Geometry check sheet. Reference: the model listing, model coordinates, mm. Round coordinates to 2 decimals unless told otherwise and drop trailing zeros. One line per item, written item: value. Start each with the question number.
1. Section check A-A (x = 225). Count the separate pieces of the cut face and the enclosed holes in it, and give its area (3 significant figures).
2. Depth check by flat-ended pin: P1, Ø4, axis at x = 245.5, z = -114, coming from the +Y side. Enter the tip coordinate at first touch or a pass-through.
3. Scan lines: probe 1 along Z at (x, y) = (234, 4.2); probe 2 along X at (y, z) = (2.5, -82.5); probe 3 along X at (y, z) = (9.2, -94.25). Record each from-to range of solid material in increasing order. Write a range as [from, to].
from build123d import *

# Parameters (mm, degrees)
SKICA1_W                 = 400
SKICA1_H                 = 225
P_IDAT_VYSUNUT_M1_DEPTH  = 10
SKICA2_R                 = 102.5
ODEBRAT_VYSUNUT_M1_DEPTH = 10
ZAOBLIT1_R               = 10
SKICA3_R                 = 4
ODEBRAT_VYSUNUT_M2_DEPTH = 10
SKICA4_R                 = 7.5
ODEBRAT_VYSUNUT_M3_DEPTH = 6
ZKOSEN_1_SIZE            = 0.5
ZKOSEN_2_SIZE            = 1
ZKOSEN_3_SIZE            = 1
SKICA5_R                 = 2
ODEBRAT_VYSUNUT_M4_DEPTH = 10
SKICA6_R                 = 2
ODEBRAT_VYSUNUT_M5_DEPTH = 10
SKICA7_R                 = 4
ODEBRAT_VYSUNUT_M6_DEPTH = 4


with BuildPart() as part:
    # Skica1 → Přidat vysunutím1 (new body)
    with BuildSketch(Plane(origin=(0, 0, 0), x_dir=(1, 0, 0), z_dir=(0, 1, 0))):
        with Locations((200, 112.5)):
            Rectangle(SKICA1_W, SKICA1_H)
    extrude(amount=P_IDAT_VYSUNUT_M1_DEPTH)

    # Skica2 → Odebrat vysunutím1 (cut)
    with BuildSketch(Plane(origin=(0, 10, 0), x_dir=(1, 0, 0), z_dir=(0, 1, 0))):
        with Locations(Location((112.5, 112.5, 0), (0, 0, 270))):
            Circle(SKICA2_R)
    extrude(amount=-ODEBRAT_VYSUNUT_M1_DEPTH, mode=Mode.SUBTRACT)

    # Zaoblit1
    zaoblit1_edges = [part.edges().sort_by_distance(p)[0] for p in [
        (0, 5, -225),
        (400, 5, -225),
        (400, 5, 0),
        (0, 5, 0),
    ]]
    fillet(zaoblit1_edges, radius=ZAOBLIT1_R)

    # Skica3 → Odebrat vysunutím2 (cut)
    with BuildSketch(Plane(origin=(0, 10, 0), x_dir=(1, 0, 0), z_dir=(0, 1, 0))):
        with Locations(Location((10, 215, 0), (0, 0, 270))):
            Circle(SKICA3_R)
        with Locations(Location((390, 215, 0), (0, 0, 270))):
            Circle(SKICA3_R)
        with Locations(Location((10, 10, 0), (0, 0, 270))):
            Circle(SKICA3_R)
        with Locations(Location((390, 10, 0), (0, 0, 270))):
            Circle(SKICA3_R)
        with Locations(Location((225, 215, 0), (0, 0, 270))):
            Circle(SKICA3_R)
        with Locations(Location((225, 10, 0), (0, 0, 270))):
            Circle(SKICA3_R)
    extrude(amount=-ODEBRAT_VYSUNUT_M2_DEPTH, mode=Mode.SUBTRACT)

    # Skica4 → Odebrat vysunutím3 (cut)
    with BuildSketch(Plane(origin=(0, 10, 0), x_dir=(1, 0, 0), z_dir=(0, 1, 0))):
        with Locations(Location((10, 215, 0), (0, 0, 270))):
            Circle(SKICA4_R)
        with Locations(Location((390, 215, 0), (0, 0, 270))):
            Circle(SKICA4_R)
        with Locations(Location((10, 10, 0), (0, 0, 270))):
            Circle(SKICA4_R)
        with Locations(Location((390, 10, 0), (0, 0, 270))):
            Circle(SKICA4_R)
        with Locations(Location((225, 215, 0), (0, 0, 270))):
            Circle(SKICA4_R)
        with Locations(Location((225, 10, 0), (0, 0, 270))):
            Circle(SKICA4_R)
    extrude(amount=-ODEBRAT_VYSUNUT_M3_DEPTH, mode=Mode.SUBTRACT)

    # Zkosení1
    zkosen_1_edges = [part.edges().sort_by_distance(p)[0] for p in [
        (225, 0, -219),
        (390, 0, -14),
        (10, 0, -14),
        (390, 0, -219),
        (225, 0, -14),
        (10, 0, -219),
        (225, 10, -222.5),
        (225, 4, -219),
        (390, 10, -17.5),
        (390, 4, -14),
        (10, 10, -17.5),
        (10, 4, -14),
        (390, 10, -222.5),
        (390, 4, -219),
        (225, 10, -17.5),
        (225, 4, -14),
        (10, 10, -222.5),
        (10, 4, -219),
    ]]
    chamfer(zkosen_1_edges, length=ZKOSEN_1_SIZE)

    # Zkosení2
    zkosen_2_edges = [part.edges().sort_by_distance(p)[0] for p in [
        (112.5, 10, -215),
        (112.5, 0, -215),
    ]]
    chamfer(zkosen_2_edges, length=ZKOSEN_2_SIZE)

    # Zkosení3
    zkosen_3_edges = [part.edges().sort_by_distance(p)[0] for p in [
        (200, 0, -225),
        (200, 10, -225),
        (0, 0, -112.5),
        (400, 0, -112.5),
        (200, 0, 0),
        (2.928932188, 0, -2.928932188),
        (2.928932188, 0, -222.071067812),
        (397.071067812, 0, -2.928932188),
        (397.071067812, 0, -222.071067812),
        (400, 10, -112.5),
        (0, 10, -112.5),
        (200, 10, 0),
        (2.928932188, 10, -2.928932188),
        (2.928932188, 10, -222.071067812),
        (397.071067812, 10, -2.928932188),
        (397.071067812, 10, -222.071067812),
    ]]
    chamfer(zkosen_3_edges, length=ZKOSEN_3_SIZE)

    # Skica5 → Odebrat vysunutím4 (cut)
    with BuildSketch(Plane(origin=(0, 10, 0), x_dir=(1, 0, 0), z_dir=(0, 1, 0))):
        with Locations(Location((352.5, 142.5, 0), (0, 0, 270))):
            Circle(SKICA5_R)
        with Locations(Location((387.5, 142.5, 0), (0, 0, 270))):
            Circle(SKICA5_R)
        with Locations(Location((387.5, 82.5, 0), (0, 0, 270))):
            Circle(SKICA5_R)
        with Locations(Location((352.5, 82.5, 0), (0, 0, 270))):
            Circle(SKICA5_R)
    extrude(amount=-ODEBRAT_VYSUNUT_M4_DEPTH, mode=Mode.SUBTRACT)

    # Skica6 → Odebrat vysunutím5 (cut)
    with BuildSketch(Plane(origin=(0, 10, 0), x_dir=(1, 0, 0), z_dir=(0, 1, 0))):
        with Locations(Location((234, 115.25, 0), (0, 0, 270))):
            Circle(SKICA6_R)
        with Locations(Location((246, 115.25, 0), (0, 0, 270))):
            Circle(SKICA6_R)
        with Locations(Location((246, 94.25, 0), (0, 0, 90))):
            Circle(SKICA6_R)
        with Locations(Location((234, 94.25, 0), (0, 0, 90))):
            Circle(SKICA6_R)
    extrude(amount=-ODEBRAT_VYSUNUT_M5_DEPTH, mode=Mode.SUBTRACT)

    # Skica7 → Odebrat vysunutím6 (cut)
    with BuildSketch(Plane(origin=(0, 10, 0), x_dir=(1, 0, 0), z_dir=(0, 1, 0))):
        with Locations(Location((234, 115.25, 0), (0, 0, 270))):
            Circle(SKICA7_R)
        with Locations(Location((246, 115.25, 0), (0, 0, 270))):
            Circle(SKICA7_R)
        with Locations(Location((234, 94.25, 0), (0, 0, 270))):
            Circle(SKICA7_R)
        with Locations(Location((246, 94.25, 0), (0, 0, 270))):
            Circle(SKICA7_R)
    extrude(amount=-ODEBRAT_VYSUNUT_M6_DEPTH, mode=Mode.SUBTRACT)


solid = part.part
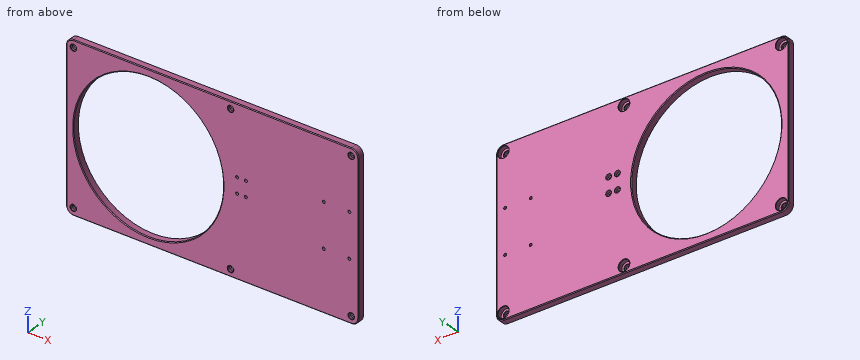
Result sheet:
1. separate pieces: 3
1. enclosed holes: 0
1. area: 2,000 mm2
2. P1: stops at y = 6
3. probe 1: z = [-225, -117.25], [-113.25, -96.25], [-92.25, 0]
3. probe 2: x = [0, 14.49], [210.51, 350.5], [354.5, 385.5], [389.5, 400]
3. probe 3: x = [0.2, 11.43], [213.57, 230], [238, 242], [250, 399.8]
